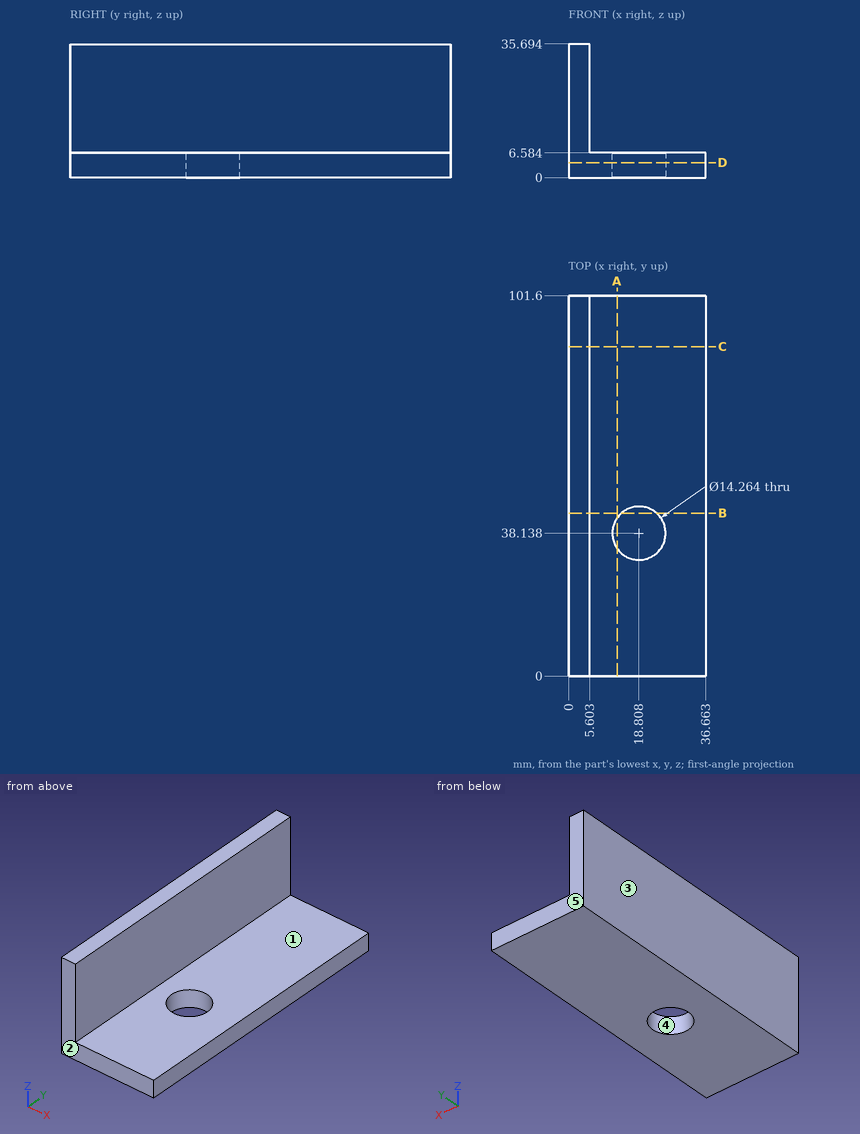
Design review of the part shown in the three views and the two pictorial views. Dimensions are in mm from the part's minimum x, y and z. A direction names the side the tool comes from. Round coordinates to 2 decimals unless told otherwise and drop trailing zeros. Loops run counter-clockwise (first coordinate to the right, second up) from the corner with the lowest first, then second, coordinate; pieces in that order, holes last.
Q1. Add section D-D on z = 4. Write out the cut boundary in (x, y).
Result sheet:
outline: (0, 0) - (36.66, 0) - (36.66, 101.6) - (0, 101.6) - close; hole circle Ø14.26 at (18.81, 38.14)
Q2. Add section B-B on y = 43.5. Write out the cut boundary in (x, z).
Result sheet:
outline: (0, 0) - (14.11, 0) - (14.11, 6.58) - (5.6, 6.58) - (5.6, 35.69) - (0, 35.69) - close; (23.51, 0) - (36.66, 0) - (36.66, 6.58) - (23.51, 6.58) - close
Q3. Machinability: for the marked faces 1 and 2, which of the approach directions +Z, -Z, +X, -X, +Y, -Y give a long, thin tool a straight path to every point of the face, cutting with its end or side? Answer none if there is none.
Result sheet:
face 1: +Z, +X, +Y, -Y
face 2: +Z, -Z, +X, -X, -Y
Q4. Insertion check: pin 1 Ø1 at (y, z) = (10, 10.5) entering from +X; pin 2 Ø15.5 at (x, y) = (17, 50.5) entering from +Z; pin 3 Ø6 at (x, z) = (9, 26.5) entering from -Y. Each pin has a flat end and moves straight along its axis. Give the tip position at first contact, or say it passes through.
Result sheet:
pin 1: stops at x = 5.6
pin 2: stops at z = 6.58
pin 3: passes through
Q5. Mouldability with a two-part tool opening along Y and no side actions: class the marked faces 3, 4 and 5 as +Y half, -Y half, draft (parallel to the pull), parting line (faces both ways), or undercut.
Result sheet:
face 3: draft
face 4: undercut
face 5: +Y half
Q6. To check wall thickness, follow line 1 along X through (y, z) = (40, 12); line 2 along Z through (x, y) = (27, 40); line 3 along Y through (x, z) = (15, 5.5). State the ranges of each line that lie inside material, in increasing order.
Result sheet:
line 1: x = 0 to 5.6
line 2: z = 0 to 6.58
line 3: y = 0 to 32.11, 44.17 to 101.6
Q7. Add section C-C on y = 88. Write out the cut boundary in (x, z).
Result sheet:
outline: (0, 0) - (36.66, 0) - (36.66, 6.58) - (5.6, 6.58) - (5.6, 35.69) - (0, 35.69) - close
Q8. Add section A-A on x = 13. Write out the cut boundary in (y, z).
Result sheet:
outline: (0, 0) - (34, 0) - (34, 6.58) - (0, 6.58) - close; (42.28, 0) - (101.6, 0) - (101.6, 6.58) - (42.28, 6.58) - close
